Print and shaded views of the part. All mm, measured from the part's lowest x, y and z. Coordinates: 2 decimals unless noted, no trailing zeros. Order: outer loops, then holes, each group sorted by start corner. A loop starts at its lowest first (then second) coordinate and runs counter-clockwise, first axis right, second up. Notation, with made-up numbers: (64, 3) -> (105, 3) arc R21 cw to (105, 18) -> close; hole circle Ø11 at (-36, -24.5). An arc over 180 degrees is marked (long way). Write item = value, one per line. Start each with the question number.
Q1. Cut at D-D, the plane z = 1.5. Give the number of separate pieces and of enclosed holes in the cut face, plus the area to 3 significant figures.
Q2. Cut at A-A, the plane x = 22. List the corners of the cut face in (y, z), plus the area to 3 significant figures.
Q3. Cut at B-B, the plane y = 11. List the corners of the cut face in (x, z) (1 decimal).
Q4. Wall check: line 1 (Y direction, x = 42, z = 1.6); line 2 (X direction, y = 5, z = 1.7) (1 decimal); line 3 (Y direction, x = 7, z = 1.1). Give the ranges that are in metal, low to high. Write a range as from..to.
Q5. Cut at C-C, the plane x = 53.5. List the corners of the cut face in (y, z).
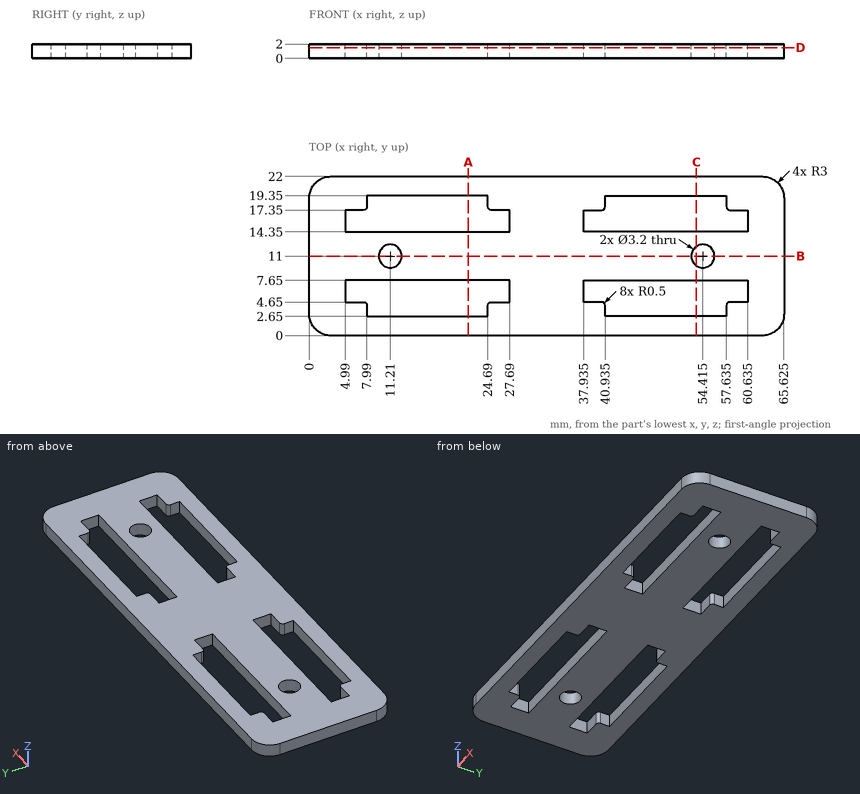
Here are the results:
q1.separate_pieces = 1
q1.enclosed_holes = 6
q1.area = 1,010 mm²
q2.outline = (0, 0) -> (2.65, 0) -> (2.65, 2) -> (0, 2) -> close; (7.65, 0) -> (14.35, 0) -> (14.35, 2) -> (7.65, 2) -> close; (19.35, 0) -> (22, 0) -> (22, 2) -> (19.35, 2) -> close
q2.area = 24.0 mm²
q3.outline = (0, 0) -> (9.6, 0) -> (9.6, 2) -> (0, 2) -> close; (12.8, 0) -> (52.8, 0) -> (52.8, 2) -> (12.8, 2) -> close; (56, 0) -> (65.6, 0) -> (65.6, 2) -> (56, 2) -> close
q4.line_1 = 0..2.65, 7.65..14.35, 19.35..22
q4.line_2 = 0..5, 27.7..37.9, 60.6..65.6
q4.line_3 = 0..4.65, 7.65..14.35, 17.35..22
q5.outline = (0, 0) -> (2.65, 0) -> (2.65, 2) -> (0, 2) -> close; (7.65, 0) -> (9.69, 0) -> (9.69, 2) -> (7.65, 2) -> close; (12.31, 0) -> (14.35, 0) -> (14.35, 2) -> (12.31, 2) -> close; (19.35, 0) -> (22, 0) -> (22, 2) -> (19.35, 2) -> close
